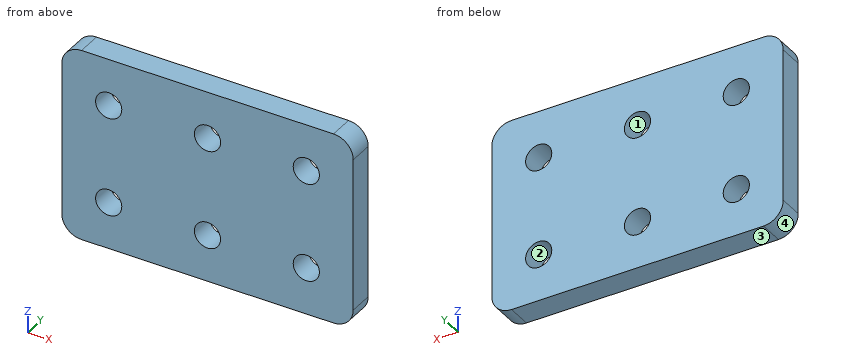
```python
from build123d import *

# Parameters (mm, degrees)
F_4_HOLE_PROFILE_SKETCH_R        = 2.65
F_4_HOLE_THICKNESS_EXTRUDE_DEPTH = 5
F_6_HOLE_EXTENSION_SKETCH_R      = 2.65
F_6_HOLE_EXTENSION_EXTRUDE_DEPTH = 5


with BuildPart() as part:
    # 4 Hole Profile Sketch → 4 Hole Thickness Extrude (new body)
    with BuildSketch(Plane(origin=(0, 0, 0), x_dir=(1, 0, 0), z_dir=(0, 1, 0))):
        with BuildLine():
            Line((-15.5, -19.5), (15.5, -19.5))
            ThreePointArc((15.5, -19.5), (18.328427125, -18.328427125), (19.5, -15.5))
            Line((19.5, -15.5), (19.5, 15.5))
            ThreePointArc((19.5, 15.5), (18.328427125, 18.328427125), (15.5, 19.5))
            Line((15.5, 19.5), (-15.5, 19.5))
            ThreePointArc((-15.5, 19.5), (-18.328427125, 18.328427125), (-19.5, 15.5))
            Line((-19.5, 15.5), (-19.5, -15.5))
            ThreePointArc((-19.5, -15.5), (-18.328427125, -18.328427125), (-15.5, -19.5))
        make_face()
        with Locations(Location((10, -10, 0), (0, 0, 270))):
            Circle(F_4_HOLE_PROFILE_SKETCH_R, mode=Mode.SUBTRACT)
        with Locations(Location((10, 10, 0), (0, 0, 270))):
            Circle(F_4_HOLE_PROFILE_SKETCH_R, mode=Mode.SUBTRACT)
        with Locations(Location((-10, -10, 0), (0, 0, 270))):
            Circle(F_4_HOLE_PROFILE_SKETCH_R, mode=Mode.SUBTRACT)
        with Locations(Location((-10, 10, 0), (0, 0, 270))):
            Circle(F_4_HOLE_PROFILE_SKETCH_R, mode=Mode.SUBTRACT)
    extrude(amount=F_4_HOLE_THICKNESS_EXTRUDE_DEPTH)

    # 6 Hole Extension Sketch → 6 Hole Extension Extrude (add)
    with BuildSketch(Plane(origin=(0, 0, 0), x_dir=(1, 0, 0), z_dir=(0, 1, 0))):
        with BuildLine():
            Line((39.5, -15.5), (39.5, 15.5))
            ThreePointArc((39.5, 15.5), (38.328427125, 18.328427125), (35.5, 19.5))
            Line((35.5, 19.5), (15.5, 19.5))
            ThreePointArc((15.5, 19.5), (18.328427125, 18.328427125), (19.5, 15.5))
            Line((19.5, 15.5), (19.5, -15.5))
            ThreePointArc((19.5, -15.5), (18.328427125, -18.328427125), (15.5, -19.5))
            Line((15.5, -19.5), (35.5, -19.5))
            ThreePointArc((35.5, -19.5), (38.328427125, -18.328427125), (39.5, -15.5))
        make_face()
        with Locations(Location((30, -10, 0), (0, 0, 270))):
            Circle(F_6_HOLE_EXTENSION_SKETCH_R, mode=Mode.SUBTRACT)
        with Locations(Location((30, 10, 0), (0, 0, 270))):
            Circle(F_6_HOLE_EXTENSION_SKETCH_R, mode=Mode.SUBTRACT)
    extrude(amount=F_6_HOLE_EXTENSION_EXTRUDE_DEPTH)


solid = part.part
```
Model file for the job. Use its own axes, mm. Face numbers are marked on the shaded views. Round coordinates to 2 decimals unless told otherwise and drop trailing zeros. Order: outer loops, then holes, each group sorted by start corner. A loop starts at its lowest first (then second) coordinate and runs counter-clockwise, first axis right, second up. Notation, with made-up numbers: M 14.25,-31 L 64.25,-31 A6 cw 64.25,-23 Z; hole C -21,74 d3. An arc over 180 degrees is marked long. Use CSV: the item, a comma, the result in double quotes.
Item 1: Saw through at D-D (x = 11). List the corners of the cut face in (y, z), plus the area to 3 significant figures.
Worked answers:
outline,"M 0,-19.5 L 5,-19.5 L 5,-12.45 L 0,-12.45 Z; M 0,-7.55 L 5,-7.55 L 5,7.55 L 0,7.55 Z; M 0,12.45 L 5,12.45 L 5,19.5 L 0,19.5 Z"
area,"146 mm²"
Item 2: Pin check, flat tip, straight feed: pin 1 (3 mm diameter, centred on x = 10, z = -10, fed in from +Y). Stop position of the tip, or through.
Worked answers:
pin 1,"through"
Item 3: Pull direction X, two halves, no side cores. Call the marked faces 1, 2, 3 and 4: released by +X, released by -X, zero draft, split by the parting line, or undercut.
Worked answers:
face 1,"undercut"
face 2,"undercut"
face 3,"zero draft"
face 4,"released by -X"
Item 4: Saw through at C-C (z = 10). List the corners of the cut face in (x, y).
Worked answers:
outline,"M -19.5,0 L -12.65,0 L -12.65,5 L -19.5,5 Z; M -7.35,0 L 7.35,0 L 7.35,5 L -7.35,5 Z; M 12.65,0 L 27.35,0 L 27.35,5 L 12.65,5 Z; M 32.65,0 L 39.5,0 L 39.5,5 L 32.65,5 Z"
Item 5: Probe probe 1 along X at (y, z) = (2.6, 10); probe 2 along Z at (x, y) = (-9, 1.5); probe 3 along Z at (x, y) = (11.5, 0.6). List the from-to ranges inside material, lowest first.
Worked answers:
probe 1,"-19.5 to -12.65, -7.35 to 7.35, 12.65 to 27.35, 32.65 to 39.5"
probe 2,"-19.5 to -12.45, -7.55 to 7.55, 12.45 to 19.5"
probe 3,"-19.5 to -12.18, -7.82 to 7.82, 12.18 to 19.5"
Item 6: Saw through at A-A (x = 30). List the corners of the cut face in (y, z), plus the area to 3 significant figures.
Worked answers:
outline,"M 0,-19.5 L 5,-19.5 L 5,-12.65 L 0,-12.65 Z; M 0,-7.35 L 5,-7.35 L 5,7.35 L 0,7.35 Z; M 0,12.65 L 5,12.65 L 5,19.5 L 0,19.5 Z"
area,"142 mm²"
Item 7: Saw through at B-B (y = 4.05). List the corners of the cut face in (x, z).
Worked answers:
outline,"M -19.5,-15.5 A4 ccw -15.5,-19.5 L 35.5,-19.5 A4 ccw 39.5,-15.5 L 39.5,15.5 A4 ccw 35.5,19.5 L -15.5,19.5 A4 ccw -19.5,15.5 Z; hole C -10,-10 d5.3; hole C -10,10 d5.3; hole C 10,-10 d5.3; hole C 10,10 d5.3; hole C 30,-10 d5.3; hole C 30,10 d5.3"
